```python
from build123d import *


with BuildPart() as f1:
    # F0 (on Front) → F1 (revolve)
    with BuildSketch(Plane.XZ):
        with BuildLine():
            Line((0, 19.8536554546), (0, 22.1536554546))
            ThreePointArc((0, 22.1536554546), (-15.665, 15.665), (-22.1536554546, 0))
            Line((-22.1536554546, 0), (-19.8536554546, 0))
            ThreePointArc((-19.8536554546, 0), (-14.0386544033, 14.0386544033), (0, 19.8536554546))
        make_face()
    revolve(axis=Axis((0, 0, 21.0036554546), (0, 0, 1)))

    # F3: F2 across plane


with BuildPart() as f2:
    # F0 (on Front) → F2 (revolve)
    with BuildSketch(Plane.XZ):
        with BuildLine():
            ThreePointArc((14.0386544033, 14.0386544033), (12.5449793362, 15.3880189876), (10.9223480336, 16.5792022831))
            Line((10.9223480336, 16.5792022831), (8.4949372388, 14.1517914883))
            Line((8.4949372388, 14.1517914883), (11.3233643635, 11.3233643635))
            Line((11.3233643635, 11.3233643635), (14.0386544033, 14.0386544033))
        make_face()
        with BuildLine():
            ThreePointArc((15.665, 15.665), (15.176552286, 16.1386712808), (14.6737888804, 16.5971193252))
            Line((14.6737888804, 16.5971193252), (13.897233047, 15.8205634919))
            Line((13.897233047, 15.8205634919), (12.0304711447, 17.6873253942))
            Line((12.0304711447, 17.6873253942), (10.9223480336, 16.5792022831))
            ThreePointArc((10.9223480336, 16.5792022831), (12.5449793362, 15.3880189876), (14.0386544033, 14.0386544033))
            Line((14.0386544033, 14.0386544033), (15.665, 15.665))
        make_face()
    revolve(axis=Axis((7.8325, 0, 7.8325), (0.7071067812, 0, 0.7071067812)))


with BuildPart() as f1_1:
    add(f1.part)
    add(f2.part.mirror(Plane.YZ), mode=Mode.SUBTRACT)

    # F4: cut F2
    add(f2.part, mode=Mode.SUBTRACT)


solid = f1_1.part
```
CAD build for the part. Positions are in the model's coordinates, mm. Coordinates: 2 decimals unless noted, no trailing zeros. Order: outer loops, then holes, each group sorted by start corner. A loop starts at its lowest first (then second) coordinate and runs counter-clockwise, first axis right, second up. Notation, with made-up numbers: M 15.5,-3.5 L 71.5,-3.5 A10 cw 71.5,10.5 Z; hole C 65,89.25 d1. An arc over 180 degrees is marked long. Write each question's results on one line, items separated by ' | '. Start each with the question number.
Q1. Pull direction Z, two halves, no side cores. Call faces 1 (the flat face through (20, 2, 0)), 2 (the flat face through (16.08, -0.06, 13.64)): +Z half, -Z half, draft (parallel to the pull), parting line (faces both ways), or undercut.
Q2. Cut at D-D (y = -16.5). List the corners of the cut face in (x, z).
Q3. Cut at B-B (y = 2). List the corners of the cut face in (x, z).
Q4. Flat gauge pins, fed straight in: P1, Ø4, axis at y = -12.5, z = 17.5, coming from the +X side; P2, Ø4, axis at x = 6, z = 4.5, coming from the +Y side; P3, Ø1, axis at x = 1.5, y = -15, coming from the +Z side. Where does each tip first touch, or does it go through?
Q5. Cut at A-A (z = 2.5). List the corners of the cut face in (x, y), then the cut area to 3 significant figures.
Q6. Drill centre lines: probe 1 along X at (y, z) = (8.5, 10); probe 2 along Y at (x, z) = (14.5, 7.75); probe 3 along X at (y, z) = (-10.5, 4.25). Where is each one in solid material? Low to high. Write a range as from..to.
Q7. Cut at C-C (x = -18.5). List the corners of the cut face in (y, z).
Found:
1) face 1: -Z half | face 2: undercut
2) outline: M -14.78,0 L -11.04,0 A11.04 cw 11.04,0 L 14.78,0 A14.78 ccw Z
3) outline: M -22.06,0 L -19.75,0 A19.75 cw -16.2,11.3 L -17.31,12.41 L -12.41,17.31 L -11.3,16.2 A19.75 cw 11.3,16.2 L 12.41,17.31 L 17.31,12.41 L 16.2,11.3 A19.75 cw 19.75,0 L 22.06,0 A22.06 ccw Z
4) P1: x = 10.5 | P2: y = 21.46 | P3: z = 16.68
5) outline: C 0,0 d44.02; hole C 0,0 d39.39 | area: 304 mm²
6) probe 1: -17.85..-14.9, 14.9..17.85 | probe 2: -14.85..-11.13, 11.13..14.85 | probe 3: -19.04..-16.31, 16.31..19.04
7) outline: M -12.19,0 L -7.21,0 A7.21 cw 7.21,0 L 12.19,0 A12.19 ccw Z
